```python
from build123d import *

# Parameters (mm, degrees)
SKETCH1_W                       = 80
SKETCH1_H                       = 13
BOSS_EXTRUDE1_DEPTH             = 13
M4X0_7_TAPPED_HOLE1_D           = 3.3
M4X0_7_TAPPED_HOLE1_CSINK_D     = 4.5
M4X0_7_TAPPED_HOLE1_CSINK_ANGLE = 90
M5X0_8_TAPPED_HOLE1_D           = 4.2
M5X0_8_TAPPED_HOLE1_CSINK_D     = 5.5
M5X0_8_TAPPED_HOLE1_CSINK_ANGLE = 90


with BuildPart() as part:
    # Sketch1 → Boss-Extrude1 (new body)
    with BuildSketch(Plane(origin=(0, 0, 0), x_dir=(1, 0, 0), z_dir=(0, 1, 0))):
        with Locations((40, 6.5)):
            Rectangle(SKETCH1_W, SKETCH1_H)
    extrude(amount=BOSS_EXTRUDE1_DEPTH)

    # M4x0.7 Tapped Hole1 (through all)
    with Locations(Plane(origin=(74.979, 13, -6.5), x_dir=(0, 0, 1), z_dir=(0, 1, 0))):
        with Locations((0, 0), (0, -14.5)):
            CounterSinkHole(M4X0_7_TAPPED_HOLE1_D / 2, M4X0_7_TAPPED_HOLE1_CSINK_D / 2, counter_sink_angle=M4X0_7_TAPPED_HOLE1_CSINK_ANGLE)

    # M5x0.8 Tapped Hole1 (through all)
    with Locations(Plane(origin=(5.067, 13, -6.5), x_dir=(0, 0, 1), z_dir=(0, 1, 0))):
        with Locations((0, 0), (0, 14.5)):
            CounterSinkHole(M5X0_8_TAPPED_HOLE1_D / 2, M5X0_8_TAPPED_HOLE1_CSINK_D / 2, counter_sink_angle=M5X0_8_TAPPED_HOLE1_CSINK_ANGLE)


solid = part.part
```
Build history of the part. All positions in model axes, mm. Round coordinates to 2 decimals unless told otherwise and drop trailing zeros. Order: outer loops, then holes, each group sorted by start corner. A loop starts at its lowest first (then second) coordinate and runs counter-clockwise, first axis right, second up. Notation, with made-up numbers: (83, 40) -> (127, 40) arc R17 ccw to (127, 49) -> close; hole circle Ø2 at (50.5, 77.5). An arc over 180 degrees is marked (long way). Answer in a Markdown table with one row per item.
1) Band-saw the part on A-A on z = -6.5. Give the cut face in (x, y), and give its area (3 significant figures).
Values:
| item | result |
|---|---|
| outline | (0, 0) -> (2.97, 0) -> (2.97, 12.35) -> (2.32, 13) -> (0, 13) -> close; (7.17, 0) -> (17.47, 0) -> (17.47, 12.35) -> (16.82, 13) -> (7.82, 13) -> (7.17, 12.35) -> close; (21.67, 0) -> (58.83, 0) -> (58.83, 12.4) -> (58.23, 13) -> (22.32, 13) -> (21.67, 12.35) -> close; (62.13, 0) -> (73.33, 0) -> (73.33, 12.4) -> (72.73, 13) -> (62.73, 13) -> (62.13, 12.4) -> close; (76.63, 0) -> (80, 0) -> (80, 13) -> (77.23, 13) -> (76.63, 12.4) -> close |
| area | 843 mm2 |
2) Wall check: L1, parallel to X at y = 6, z = -6.5; L2, parallel to X at y = 9.75, z = -5.5; L3, parallel to X at y = 8.5, z = -4.75. Give the ranges that are in metal, low to high.
Values:
| item | result |
|---|---|
| L1 | 0 to 2.97, 7.17 to 17.47, 21.67 to 58.83, 62.13 to 73.33, 76.63 to 80 |
| L2 | 0 to 3.22, 6.91 to 17.72, 21.41 to 59.17, 61.79 to 73.67, 76.29 to 80 |
| L3 | 0 to 3.91, 6.23 to 18.41, 20.73 to 80 |
3) Band-saw the part on B-B on y = 10. Give the cut face in (x, z).
Values:
| item | result |
|---|---|
| outline | (0, -13) -> (80, -13) -> (80, 0) -> (0, 0) -> close; hole circle Ø4.2 at (5.07, -6.5); hole circle Ø4.2 at (19.57, -6.5); hole circle Ø3.3 at (60.48, -6.5); hole circle Ø3.3 at (74.98, -6.5) |
4) Pin check, flat tip, straight feed: P1, Ø5, axis at x = 19.567, z = -6.5, coming from the +Y side. Stop position of the tip, or through.
Values:
| item | result |
|---|---|
| P1 | y = 12.75 |
5) Mould opens along X. For faces 1 (the flat face through (80, 6, -6)), 2 (the flat face through (39, 6, 0)), 3 (the flat face through (0, 6, -6)), 4 (the cylindrical face through (73.37, 6.11, -6.14)) say: released by +X, released by -X, zero draft, split by the parting line, or undercut.
Values:
| item | result |
|---|---|
| face 1 | released by +X |
| face 2 | zero draft |
| face 3 | released by -X |
| face 4 | undercut |
